Input: part model. Units: mm. Frame: model coordinates. A direction names the side the tool comes from. Coordinates: 2 decimals unless noted, no trailing zeros. Loops run counter-clockwise (first coordinate to the right, second up) from the corner with the lowest first, then second, coordinate; pieces in that order, holes last.
(1) Section B-B, the plane x = -8. Return loops of the section in (y, z).
(2) Section A-A, the plane z = 17.5. Return loops of the section in (x, y).
(3) Section C-C, the plane y = -12. Return loops of the section in (x, z), then the cut area to 3 significant figures.
(4) Line query: L1, parallel to X at y = 15.5, z = 16.75; L2, parallel to Y at x = -22, z = 17.25; L3, parallel to Z at x = 19, y = -14. Output: solid intervals per line, ascending.
(5) Contact query for a flat-ended pin moving along its axis: P1, Ø1.5, axis at x = -2, y = 2, coming from the +Z side. Output: stop coordinate, or through.
(6) Set-up query: faces 1 (the face through (-23, 12.603, 15)), 2 (the face through (-20.74, 15, 15)), 3 (the face through (-23, -15, 25)). Return all of +Z, -Z, +X, -X, +Y, -Y with unobstructed straight access to the full face (end or side cutting, diameter ignored); none if empty.
(7) Mould query, pull axis X, two halves, no side actions, for faces 4 (the face through (25, 0, 4)), 5 (the face through (23, 15, 25)), 6 (the face through (20.74, 15, 15)). Classes: released by +X, released by -X, zero draft, split by the parting line, or undercut.
```python
from build123d import *

# Parameters (mm, degrees)
F0_W     = 4.2595966585
F0_H     = 4.2287140257
F1_DEPTH = 5
F2_DEPTH = 25


with BuildPart() as f1:
    # F0 (on Top) → F1 (new body)
    with BuildSketch(Plane.XY):
        with Locations((-22.8702016707, 14.7173251896)):
            Rectangle(F0_W, F0_H)
        Polygon((20.7404033415, 16.8316822024), (-20.7404033415, 16.8316822024), (-20.7404033415, 12.6029681767), (-25, 12.6029681767), (-25, -12.6029681767), (-20.7404033415, -12.6029681767), (-20.7404033415, -16.8316822024), (20.7404033415, -16.8316822024), (20.7404033415, -12.6029681767), (25, -12.6029681767), (25, 12.6029681767), (20.7404033415, 12.6029681767), align=None)
        with Locations((22.8702016707, 14.7173251896)):
            Rectangle(F0_W, F0_H)
        with Locations((-22.8702016707, -14.7173251896)):
            Rectangle(F0_W, F0_H)
        with Locations((22.8702016707, -14.7173251896)):
            Rectangle(F0_W, F0_H)
    extrude(amount=F1_DEPTH)

    # F0 (on Top) → F2 (join)
    with BuildSketch(Plane.XY):
        with Locations((22.8702016707, 14.7173251896)):
            Rectangle(F0_W, F0_H)
        with Locations((22.8702016707, -14.7173251896)):
            Rectangle(F0_W, F0_H)
        with Locations((-22.8702016707, -14.7173251896)):
            Rectangle(F0_W, F0_H)
        with Locations((-22.8702016707, 14.7173251896)):
            Rectangle(F0_W, F0_H)
    extrude(amount=F2_DEPTH)


solid = f1.part
```
Report:
1. outline: (-16.83, 0) - (16.83, 0) - (16.83, 5) - (-16.83, 5) - close
2. outline: (-25, -16.83) - (-20.74, -16.83) - (-20.74, -12.6) - (-25, -12.6) - close; (-25, 12.6) - (-20.74, 12.6) - (-20.74, 16.83) - (-25, 16.83) - close; (20.74, -16.83) - (25, -16.83) - (25, -12.6) - (20.74, -12.6) - close; (20.74, 12.6) - (25, 12.6) - (25, 16.83) - (20.74, 16.83) - close
3. outline: (-25, 0) - (25, 0) - (25, 5) - (-25, 5) - close
3. area: 250 mm2
4. L1: x = -25 to -20.74, 20.74 to 25
4. L2: y = -16.83 to -12.6, 12.6 to 16.83
4. L3: z = 0 to 5
5. P1: stops at z = 5
6. face 1: +Z, +X, -X
6. face 2: +Z, +Y, -Y
6. face 3: +Z, +X, -X, +Y, -Y
7. face 4: released by +X
7. face 5: zero draft
7. face 6: undercut
